```python
from build123d import *

# Parameters (mm, degrees)
BOSS_EXTRUDE1_DEPTH     = 1.5875
F_1_4_CLEARANCE_HOLE1_D = 6.5278
FILLET1_R               = 6.35


with BuildPart() as part:
    # Sketch2 → Boss-Extrude1 (new, symmetric)
    with BuildSketch(Plane(origin=(0, 0, 0), x_dir=(0, 0, -1), z_dir=(1, 0, 0))):
        Polygon((4.639999991, 33.98455115), (4.639999991, -33.98455115), (24.959999991, -41.373642063), (24.959999991, 41.373642063), align=None)
    extrude(amount=BOSS_EXTRUDE1_DEPTH, both=True)

    # 1/4 Clearance Hole1 (through all)
    with Locations(Plane(origin=(1.5875, 0, 0), x_dir=(0, 0, -1), z_dir=(1, 0, 0))):
        with Locations((14.799999991, 0), (14.799999991, 25.4), (14.799999991, -25.4)):
            Hole(F_1_4_CLEARANCE_HOLE1_D / 2)

    # Fillet1
    fillet1_edges = [part.edges().sort_by_distance(p)[0] for p in [
        (0, 41.373642063, -24.959999991),
        (0, -41.373642063, -24.959999991),
        (0, -33.98455115, -4.639999991),
        (0, 33.98455115, -4.639999991),
    ]]
    fillet(fillet1_edges, radius=FILLET1_R)


solid = part.part
```
The listing builds one solid part. Answer for the finished solid, in the listing's coordinates (mm). Coordinates: 2 decimals unless noted, no trailing zeros. Write each loop counter-clockwise with the first axis right and the second up, starting at its lowest first coordinate (ties: lowest second). Pieces come first, ordered by that corner, then holes. Notation, with made-up numbers: (14.25, -27.75) - (18.25, -27.75) arc R18 cw to (18.25, -22.75) - close; hole circle Ø5 at (-5, 46). An arc over 180 degrees is marked (long way). Return JSON: item names as keys, results as strings. Group by question number.
Q1. The part is cut by section C-C on z = -14.5. Write down the section's boundary in (x, y), and give its area (3 significant figures).
Q2. The part is cut by section B-B on y = 0. Write down the section's boundary in (x, z), and give its area (3 significant figures).
Q3. Find the intervals of material crossed by line 1 along Y through (x, z) = (0.95, -12.75); line 2 along Y through (x, z) = (0.3, -14.8); line 3 along Z through (x, y) = (-0.5, -26.5), in increasing order. Write a range as [from, to].
Q4. A flat-ended cylindrical pin translates along its axis: pin 1 Ø4 at (y, z) = (25.4, -14.8) entering from +X. Find the tip coordinate at first contact, or state that the pin passes through.
Q5. The part is cut by section D-D on z = -6.5. Write down the section's boundary in (x, y).
Q6. For a pull along Z with two mould halves and no side action, classify faces 1 (the cylindrical face through (0.02, -37.56, -22.18)), 2 (the flat face through (0, 0, -24.96)), 3 (the cylindrical face through (-0.022, -3.186, -15.508)) as +Z half, -Z half, draft (parallel to the pull), parting line (faces both ways), or undercut.
Q7. The part is cut by section A-A on x = 0.3. Write down the section's boundary in (y, z), and give its area (3 significant figures).
Evaluation:
{
 "1": {"outline": "(-1.59, -37.57) - (1.59, -37.57) - (1.59, -28.65) - (-1.59, -28.65) - close; (-1.59, -22.15) - (1.59, -22.15) - (1.59, -3.25) - (-1.59, -3.25) - close; (-1.59, 3.25) - (1.59, 3.25) - (1.59, 22.15) - (-1.59, 22.15) - close; (-1.59, 28.65) - (1.59, 28.65) - (1.59, 37.57) - (-1.59, 37.57) - close", "area": "177 mm2"},
 "2": {"outline": "(-1.59, -24.96) - (1.59, -24.96) - (1.59, -18.06) - (-1.59, -18.06) - close; (-1.59, -11.54) - (1.59, -11.54) - (1.59, -4.64) - (-1.59, -4.64) - close", "area": "43.8 mm2"},
 "3": {"line 1": "y = [-36.93, -27.94], [-22.86, -2.54], [2.54, 22.86], [27.94, 36.93]", "line 2": "y = [-37.68, -28.66], [-22.14, -3.26], [3.26, 22.14], [28.66, 37.68]", "line 3": "z = [-24.96, -17.87], [-11.73, -4.64]"},
 "4": {"pin 1": "passes through"},
 "5": {"outline": "(-1.59, -34.03) - (1.59, -34.03) - (1.59, 34.03) - (-1.59, 34.03) - close"},
 "6": {"face 1": "parting line", "face 2": "-Z half", "face 3": "undercut"},
 "7": {"outline": "(-38.28, -16.44) arc R6.35 ccw to (-32.31, -24.96) - (32.31, -24.96) arc R6.35 ccw to (38.28, -16.44) - (35.5, -8.82) arc R6.35 ccw to (29.54, -4.64) - (-29.54, -4.64) arc R6.35 ccw to (-35.5, -8.82) - close; hole circle Ø6.53 at (-25.4, -14.8); hole circle Ø6.53 at (0, -14.8); hole circle Ø6.53 at (25.4, -14.8)", "area": "1,390 mm2"}
}
